Here's the drawing with two shaded views (mm, measured from the low corner). I have some questions. Round coordinates to 2 decimals unless told otherwise and drop trailing zeros. Loops run counter-clockwise (first coordinate to the right, second up) from the corner with the lowest first, then second, coordinate; pieces in that order, holes last.
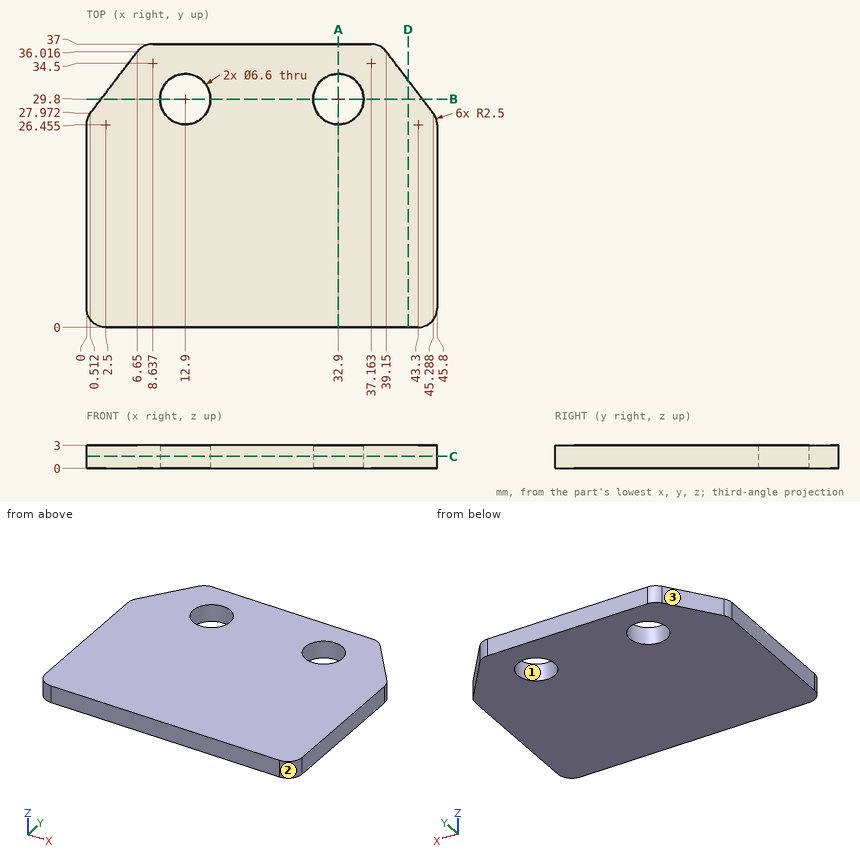
Item 1: If we section it at C-C, the plane z = 1.55: Count the separate pieces of the cut face and the enclosed holes in it, then the cut area to 3 significant figures.
Results list:
separate pieces: 1
enclosed holes: 2
area: 1,550 mm2
Item 2: If we section it at D-D, the plane x = 42: Please give me the cut outline in (y, z).
Results list:
outline: (0, 0) - (32.28, 0) - (32.28, 3) - (0, 3) - close
Item 3: We'd pull the mould along X, two halves only. Please class the marked faces 1, 2 and 3: released by +X, released by -X, zero draft, split by the parting line, or undercut.
Results list:
face 1: undercut
face 2: released by +X
face 3: released by -X
Item 4: If we section it at B-B, the plane y = 29.8: Please give me the cut outline in (x, z).
Results list:
outline: (1.91, 0) - (9.6, 0) - (9.6, 3) - (1.91, 3) - close; (16.2, 0) - (29.6, 0) - (29.6, 3) - (16.2, 3) - close; (36.2, 0) - (43.89, 0) - (43.89, 3) - (36.2, 3) - close
Item 5: If we section it at A-A, the plane x = 32.9: Please give me the cut outline in (y, z).
Results list:
outline: (0, 0) - (26.5, 0) - (26.5, 3) - (0, 3) - close; (33.1, 0) - (37, 0) - (37, 3) - (33.1, 3) - close
Item 6: If I drill on line 1 along X through (y, z) = (29.8, 1.8); line 2 along Y through (x, z) = (32.9, 1.8); line 3 along Y through (x, z) = (31, 1.7), over which ranges is the centre line in solid material (lowest first)?
Results list:
line 1: x = 1.91 to 9.6, 16.2 to 29.6, 36.2 to 43.89
line 2: y = 0 to 26.5, 33.1 to 37
line 3: y = 0 to 27.1, 32.5 to 37
